Read the model definition and answer for the solid it produces. Units are mm, in the model's axes. Face numbers are marked on the shaded views. Give positions to 0.01 mm unless a question says otherwise; leave off trailing zeros. Write each loop counter-clockwise with the first axis right and the second up, starting at its lowest first coordinate (ties: lowest second). Pieces come first, ordered by that corner, then holes. Notation, with made-up numbers: (-26, 48) -> (27, 48) arc R31 cw to (27, 76) -> close; hole circle Ø9 at (45.25, 40.25). An arc over 180 degrees is marked (long way). Use a Markdown table: item, result.
Solid Edge part; units mm, degrees
sketch "Sketch1" plane through (0, 0, 0) normal (0, 0, 1) x (1, 0, 0)
  arc A0 (0, 5.6) -> (0.6, 5) centre (0.6, 5.6) ccw
  line L0 (0.6, 5) -> (10.4, 5)
  arc A1 (10.4, 5) -> (11, 5.6) centre (10.4, 5.6) ccw
  line L1 (11, 5.6) -> (11, 8.65)
  arc A2 (11, 8.65) -> (10.8, 8.85) centre (10.8, 8.65) ccw
  line L2 (10.8, 8.85) -> (8.2743, 8.85)
  arc A3 (8.2743, 8.85) -> (2.7257, 8.85) centre (5.5, 11.1) cw
  line L3 (2.7257, 8.85) -> (0.2, 8.85)
  arc A4 (0.2, 8.85) -> (0, 8.65) centre (0.2, 8.65) ccw
  line L4 (0, 8.65) -> (0, 5.6)
revolve "RevolvedProtrusion1" add sketch "Sketch1" angle 360 about axis through (10.4, 0, 0) along (-1, 0, 0)
properties material "Steel"
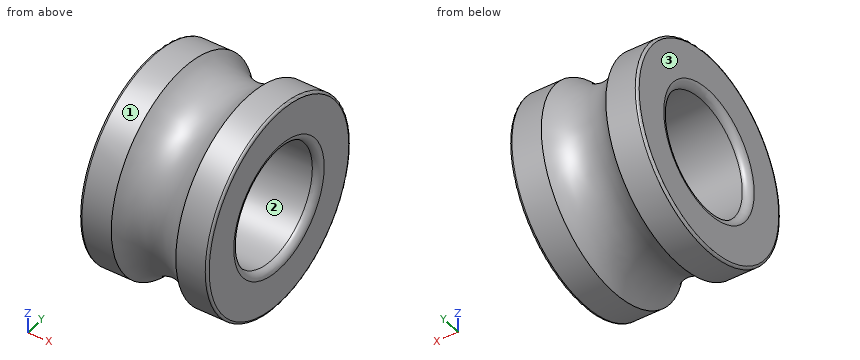
Item 1: Straight lines are drawn through the part: line 1 along Z through (x, y) = (8.5, 0); line 2 along X through (y, z) = (-1.75, -5.25); line 3 along Y through (x, z) = (3.75, 0). For each, find the intervals that lie inside material, in ascending order. Write a range as [from, to].
Return value:
| item | result |
|---|---|
| line 1 | [-8.85, -5], [5, 8.85] |
| line 2 | [0, 11] |
| line 3 | [-7.99, -5], [5, 7.99] |
Item 2: For a pull along Y with two mould halves and no side action, classify the marked faces 1, 2 and 3 as +Y half, -Y half, draft (parallel to the pull), parting line (faces both ways), or undercut.
Return value:
| item | result |
|---|---|
| face 1 | parting line |
| face 2 | undercut |
| face 3 | draft |
Item 3: Each of these flat-tipped pins is pushed along its axis until it touches: P1, Ø2, axis at x = 5, y = -4.5, coming from the +Z side; P2, Ø1.5, axis at x = 3.5, z = -2, coming from the -Y side; P3, Ø4, axis at x = 5, y = -3.5, coming from the -Z side. Where does it stop, or does it pass through?
Return value:
| item | result |
|---|---|
| P1 | z = 6.76 |
| P2 | y = -8.61 |
| P3 | z = -7.95 |
Item 4: A cutting plane is placed at A-A (z = 0). Give the vertices of the cut face in (x, y), then the cut area to 3 significant figures.
Return value:
| item | result |
|---|---|
| outline | (0, -8.65) arc R0.2 ccw to (0.2, -8.85) -> (2.73, -8.85) arc R3.57 cw to (8.27, -8.85) -> (10.8, -8.85) arc R0.2 ccw to (11, -8.65) -> (11, -5.6) arc R0.6 ccw to (10.4, -5) -> (0.6, -5) arc R0.6 ccw to (0, -5.6) -> close; (0, 5.6) arc R0.6 ccw to (0.6, 5) -> (10.4, 5) arc R0.6 ccw to (11, 5.6) -> (11, 8.65) arc R0.2 ccw to (10.8, 8.85) -> (8.27, 8.85) arc R3.57 cw to (2.73, 8.85) -> (0.2, 8.85) arc R0.2 ccw to (0, 8.65) -> close |
| area | 74.1 mm^2 |
Item 5: A cutting plane is placed at C-C (x = 5). Give the vertices of the cut face in (y, z).
Return value:
| item | result |
|---|---|
| outline | circle Ø15.13 at (0, 0); hole circle Ø10 at (0, 0) |
